Can you work these out from the drawing? Everything is in mm from the part's minimum corner. A direction names the side the tool comes from. Coordinates: 2 decimals unless noted, no trailing zeros. Loops run counter-clockwise (first coordinate to the right, second up) from the corner with the lowest first, then second, coordinate; pieces in that order, holes last.
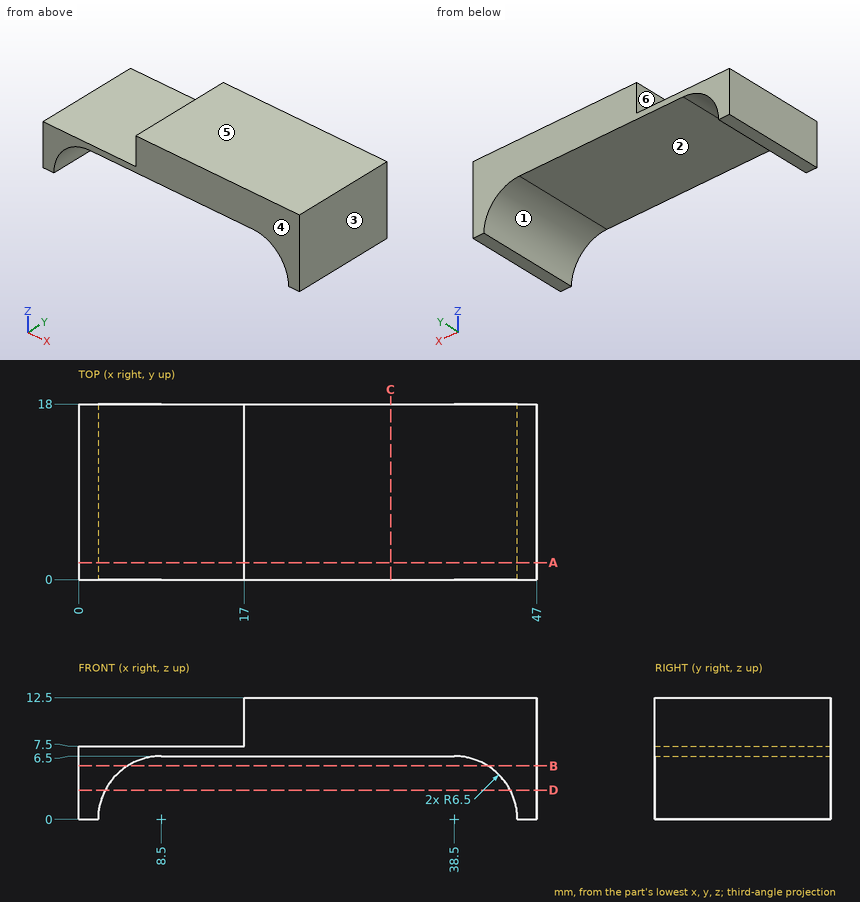
1) If I drill on L1, parallel to X at y = 1, z = 12; L2, parallel to Z at x = 34, y = 10.5; L3, parallel to X at y = 7.5, z = 2, over which ranges is the centre line in solid material (lowest first)?
2) Imagine slicing it at D-D on z = 3. List the corners of the cut face in (x, y) for me, plus the area to 3 significant figures.
3) We'd pull the mould along X, two halves only. Please class the marked faces 1, 2, 3 and 4: released by +X, released by -X, zero draft, split by the parting line, or undercut.
4) For the marked faces 5 and 6, which set-ups out of +Z, -Z, +X, -X, +Y, -Y let a thin tool reach every point of the face, with its end or its side?
5) Imagine slicing it at A-A on y = 1.75. List the corners of the cut face in (x, z) for me, plus the area to 3 significant figures.
6) Imagine slicing it at C-C on x = 32. List the corners of the cut face in (y, z) for me.
7) Will these pins go through, and if not, where does the flat tip stop? pin 1 (1 mm diameter, centred on x = 10.5, y = 13, fed in from -Z); pin 2 (5 mm diameter, centred on x = 5.5, y = 8, fed in from +Z); pin 3 (3 mm diameter, centred on x = 13, z = 9.5, fed in from +Y); pin 4 (2.5 mm diameter, centred on y = 10, z = 10, fed in from -X).
8) Imagine slicing it at B-B on z = 5.5. List the corners of the cut face in (x, y) for me, plus the area to 3 significant figures.
Solved:
1. L1: x = 17 to 47
1. L2: z = 6.5 to 12.5
1. L3: x = 0 to 2.32, 44.68 to 47
2. outline: (0, 0) - (2.73, 0) - (2.73, 18) - (0, 18) - close; (44.27, 0) - (47, 0) - (47, 18) - (44.27, 18) - close
2. area: 98.4 mm2
3. face 1: undercut
3. face 2: undercut
3. face 3: released by +X
3. face 4: zero draft
4. face 5: +Z, +X, -X, +Y, -Y
4. face 6: +Z, -X, +Y, -Y
5. outline: (0, 0) - (2, 0) arc R6.5 cw to (8.5, 6.5) - (38.5, 6.5) arc R6.5 cw to (45, 0) - (47, 0) - (47, 12.5) - (17, 12.5) - (17, 7.5) - (0, 7.5) - close
5. area: 241 mm2
6. outline: (0, 6.5) - (18, 6.5) - (18, 12.5) - (0, 12.5) - close
7. pin 1: stops at z = 6.5
7. pin 2: stops at z = 7.5
7. pin 3: passes through
7. pin 4: stops at x = 17
8. outline: (0, 0) - (5.04, 0) - (5.04, 18) - (0, 18) - close; (41.96, 0) - (47, 0) - (47, 18) - (41.96, 18) - close
8. area: 181 mm2
